```python
from build123d import *

# Parameters (mm, degrees)
SKETCH1_W           = 130
SKETCH1_H           = 80
BOSS_EXTRUDE1_DEPTH = 3.2
SKETCH2_W           = 14.444444444
SKETCH2_H           = 3.2
SKETCH2_W_2         = 3.2
SKETCH2_H_2         = 13.333333334
SKETCH2_H_3         = 13.333333333
CUT_EXTRUDE1_DEPTH  = 153.676913775
MOVE_FACE1_BY       = 0.1
MOVE_FACE1_2_BY     = 0.1
MOVE_FACE1_3_BY     = 0.1
MOVE_FACE1_4_BY     = 0.1
MOVE_FACE1_5_BY     = 0.1
MOVE_FACE1_6_BY     = 0.1
MOVE_FACE1_7_BY     = 0.1
MOVE_FACE1_8_BY     = 0.1
MOVE_FACE1_9_BY     = 0.1
MOVE_FACE1_10_BY    = 0.1
MOVE_FACE1_11_BY    = 0.1
MOVE_FACE1_12_BY    = 0.1
MOVE_FACE1_13_BY    = 0.1
MOVE_FACE1_14_BY    = 0.1
MOVE_FACE1_15_BY    = 0.1
MOVE_FACE1_16_BY    = 0.1
MOVE_FACE1_17_BY    = 0.1
MOVE_FACE1_18_BY    = 0.1
CUT_EXTRUDE2_REACH  = 154.677
SKETCH3_R           = 1.7


with BuildPart() as part:
    # Sketch1 → Boss-Extrude1 (new body)
    with BuildSketch(Plane.XY):
        with Locations((65, 40)):
            Rectangle(SKETCH1_W, SKETCH1_H)
    extrude(amount=BOSS_EXTRUDE1_DEPTH)

    # Sketch2 → Cut-Extrude1 (cut, through all)
    with BuildSketch(Plane.XY.offset(3.2)):
        with Locations((7.222222222, 1.6)):
            Rectangle(SKETCH2_W, SKETCH2_H)
        with Locations((36.111111111, 1.6)):
            Rectangle(SKETCH2_W, SKETCH2_H)
        with Locations((65, 1.6)):
            Rectangle(SKETCH2_W, SKETCH2_H)
        with Locations((93.888888889, 1.6)):
            Rectangle(SKETCH2_W, SKETCH2_H)
        Polygon((115.555555556, 0), (115.555555556, 3.2), (126.8, 3.2), (126.8, 13.333333333), (130, 13.333333333), (130, 0), align=None)
        with Locations((1.6, 20)):
            Rectangle(SKETCH2_W_2, SKETCH2_H_2)
        with Locations((1.6, 46.666666667)):
            Rectangle(SKETCH2_W_2, SKETCH2_H_3)
        with Locations((1.6, 73.333333334)):
            Rectangle(SKETCH2_W_2, SKETCH2_H_3)
        with Locations((128.4, 33.333333334)):
            Rectangle(SKETCH2_W_2, SKETCH2_H_3)
        with Locations((128.4, 60)):
            Rectangle(SKETCH2_W_2, SKETCH2_H_2)
    extrude(amount=-CUT_EXTRUDE1_DEPTH, mode=Mode.SUBTRACT)

    # Move Face1: a face moved inward by 0.1
    extrude(part.faces().sort_by_distance((128.4, 53.333333333, 1.6))[0], amount=MOVE_FACE1_BY, dir=(0, -1, 0), mode=Mode.SUBTRACT)

    # Move Face1 2: a face moved inward by 0.1
    extrude(part.faces().sort_by_distance((128.4, 26.666666667, 1.6))[0], amount=MOVE_FACE1_2_BY, dir=(0, -1, 0), mode=Mode.SUBTRACT)

    # Move Face1 3: a face moved inward by 0.1
    extrude(part.faces().sort_by_distance((128.4, 13.333333333, 1.6))[0], amount=MOVE_FACE1_3_BY, dir=(0, 1, 0), mode=Mode.SUBTRACT)

    # Move Face1 4: a face moved inward by 0.1
    extrude(part.faces().sort_by_distance((128.4, 40, 1.6))[0], amount=MOVE_FACE1_4_BY, dir=(0, 1, 0), mode=Mode.SUBTRACT)

    # Move Face1 5: a face moved inward by 0.1
    extrude(part.faces().sort_by_distance((128.4, 66.666666667, 1.6))[0], amount=MOVE_FACE1_5_BY, dir=(0, 1, 0), mode=Mode.SUBTRACT)

    # Move Face1 6: a face moved inward by 0.1
    extrude(part.faces().sort_by_distance((115.555555556, 1.6, 1.6))[0], amount=MOVE_FACE1_6_BY, dir=(-1, 0, 0), mode=Mode.SUBTRACT)

    # Move Face1 7: a face moved inward by 0.1
    extrude(part.faces().sort_by_distance((86.666666667, 1.6, 1.6))[0], amount=MOVE_FACE1_7_BY, dir=(-1, 0, 0), mode=Mode.SUBTRACT)

    # Move Face1 8: a face moved inward by 0.1
    extrude(part.faces().sort_by_distance((57.777777778, 1.6, 1.6))[0], amount=MOVE_FACE1_8_BY, dir=(-1, 0, 0), mode=Mode.SUBTRACT)

    # Move Face1 9: a face moved inward by 0.1
    extrude(part.faces().sort_by_distance((28.888888889, 1.6, 1.6))[0], amount=MOVE_FACE1_9_BY, dir=(-1, 0, 0), mode=Mode.SUBTRACT)

    # Move Face1 10: a face moved inward by 0.1
    extrude(part.faces().sort_by_distance((14.444444444, 1.6, 1.6))[0], amount=MOVE_FACE1_10_BY, dir=(1, 0, 0), mode=Mode.SUBTRACT)

    # Move Face1 11: a face moved inward by 0.1
    extrude(part.faces().sort_by_distance((43.333333333, 1.6, 1.6))[0], amount=MOVE_FACE1_11_BY, dir=(1, 0, 0), mode=Mode.SUBTRACT)

    # Move Face1 12: a face moved inward by 0.1
    extrude(part.faces().sort_by_distance((72.222222222, 1.6, 1.6))[0], amount=MOVE_FACE1_12_BY, dir=(1, 0, 0), mode=Mode.SUBTRACT)

    # Move Face1 13: a face moved inward by 0.1
    extrude(part.faces().sort_by_distance((101.111111111, 1.6, 1.6))[0], amount=MOVE_FACE1_13_BY, dir=(1, 0, 0), mode=Mode.SUBTRACT)

    # Move Face1 14: a face moved inward by 0.1
    extrude(part.faces().sort_by_distance((1.6, 26.666666667, 1.6))[0], amount=MOVE_FACE1_14_BY, dir=(0, 1, 0), mode=Mode.SUBTRACT)

    # Move Face1 15: a face moved inward by 0.1
    extrude(part.faces().sort_by_distance((1.6, 13.333333333, 1.6))[0], amount=MOVE_FACE1_15_BY, dir=(0, -1, 0), mode=Mode.SUBTRACT)

    # Move Face1 16: a face moved inward by 0.1
    extrude(part.faces().sort_by_distance((1.6, 40, 1.6))[0], amount=MOVE_FACE1_16_BY, dir=(0, -1, 0), mode=Mode.SUBTRACT)

    # Move Face1 17: a face moved inward by 0.1
    extrude(part.faces().sort_by_distance((1.6, 53.333333333, 1.6))[0], amount=MOVE_FACE1_17_BY, dir=(0, 1, 0), mode=Mode.SUBTRACT)

    # Move Face1 18: a face moved inward by 0.1
    extrude(part.faces().sort_by_distance((1.6, 66.666666667, 1.6))[0], amount=MOVE_FACE1_18_BY, dir=(0, -1, 0), mode=Mode.SUBTRACT)

    # Sketch3 → Cut-Extrude2 (cut, up to next)
    with BuildSketch(Plane.XY.offset(3.2), mode=Mode.PRIVATE) as cut_extrude2_sk1:
        with Locations((15.2, 74.5)):
            Circle(SKETCH3_R)
    cut_extrude2_tool1 = extrude(cut_extrude2_sk1.sketch, amount=-CUT_EXTRUDE2_REACH, mode=Mode.PRIVATE) & part.part
    # Sketch3 → Cut-Extrude2 (cut, up to next)
    with BuildSketch(Plane.XY.offset(3.2), mode=Mode.PRIVATE) as cut_extrude2_sk2:
        with Locations(Location((114.8, 74.5, 0), (0, 0, 180))):
            Circle(SKETCH3_R)
    cut_extrude2_tool2 = extrude(cut_extrude2_sk2.sketch, amount=-CUT_EXTRUDE2_REACH, mode=Mode.PRIVATE) & part.part
    add(cut_extrude2_tool1.solids().sort_by_distance((15.2, 74.5, 3.2))[0], mode=Mode.SUBTRACT)
    add(cut_extrude2_tool2.solids().sort_by_distance((114.8, 74.5, 3.2))[0], mode=Mode.SUBTRACT)


solid = part.part
```
Geometry: final body of the model. Coordinates: model frame, mm. A direction names the side the tool comes from. Coordinates: 2 decimals unless noted, no trailing zeros. Order: outer loops, then holes, each group sorted by start corner. A loop starts at its lowest first (then second) coordinate and runs counter-clockwise, first axis right, second up. Notation, with made-up numbers: (40.5, -19.75) - (68.5, -19.75) arc R10 ccw to (68.5, -8.75) - close; hole circle Ø8 at (68.25, 28). An arc over 180 degrees is marked (long way). Return JSON: item names as keys, results as strings. Group by question number.
1. Material intervals for line 1 along X through (y, z) = (74.5, 1.35); line 2 along Y through (x, z) = (114.8, 2.25); line 3 along X through (y, z) = (28.5, 0.8), sorted ascending. Write a range as [from, to].
2. Pin query (flat end, axial travel): pin 1 (2 mm diameter, centred on x = 15.2, y = 74.5, fed in from -Z); pin 2 (1.6 mm diameter, centred on y = 2, z = 2, fed in from -X); pin 3 (1 mm diameter, centred on y = 35, z = 1.5, fed in from +X); pin 4 (12 mm diameter, centred on x = 82, y = 51, fed in from -Z). Return the tip coordinate at first contact, or that it passes through.
3. Cut plane B-B (x = 65). Output: boundary loops of the cut face in (y, z).
4. Pull-direction query (X, two-part tool) for faces 1 (the face through (36, 3.2, 2)), 2 (the face through (126.8, 33, 2)), 3 (the face through (128, 66.767, 2)), 4 (the face through (116.05, 73.35, 1.62)); classes: pulls with the +X half, pulls with the -X half, needs draft (parallel to the pull), parting line crosses it, or undercut.
5. Cut plane C-C (z = 1.1). Count the separate pieces of the cut face and the enclosed holes in it, plus the area to 3 significant figures.
6. Cut plane A-A (y = 74.5). Output: boundary loops of the cut face in (x, z).
7. Set-up query: faces 5 (the face through (65, 3.2, 2)), 6 (the face through (128, 13.433, 2)), 7 (the face through (2, 53.433, 2)). Return all of +Z, -Z, +X, -X, +Y, -Y with unobstructed straight access to the full face (end or side cutting, diameter ignored); none if empty.
Resolved:
{
 "1": {"line 1": "x = [3.2, 13.5], [16.9, 113.1], [116.5, 130]", "line 2": "y = [0, 72.8], [76.2, 80]", "line 3": "x = [0, 126.8]"},
 "2": {"pin 1": "passes through", "pin 2": "stops at x = 14.54", "pin 3": "stops at x = 126.8", "pin 4": "stops at z = 0"},
 "3": {"outline": "(3.2, 0) - (80, 0) - (80, 3.2) - (3.2, 3.2) - close"},
 "4": {"face 1": "undercut", "face 2": "pulls with the +X half", "face 3": "needs draft", "face 4": "undercut"},
 "5": {"separate pieces": "1", "enclosed holes": "2", "area": "9,900 mm²"},
 "6": {"outline": "(3.2, 0) - (13.5, 0) - (13.5, 3.2) - (3.2, 3.2) - close; (16.9, 0) - (113.1, 0) - (113.1, 3.2) - (16.9, 3.2) - close; (116.5, 0) - (130, 0) - (130, 3.2) - (116.5, 3.2) - close"},
 "7": {"face 5": "+Z, -Z, -Y", "face 6": "+Z, -Z, +X, -Y", "face 7": "+Z, -Z, -X"}
}
